```python
from build123d import *

# Parameters (mm, degrees)
ESQUISSE1_W              = 28
ESQUISSE1_H              = 28
BOSS_EXTRU_1_DEPTH       = 4
COQUE1_T                 = 1
ENL_V_MAT_EXTRU_1_REACH  = 43.449
ESQUISSE2_W              = 25
ESQUISSE2_H              = 15
CONG_1_R                 = 4
CONG_3_R                 = 1
ENL_V_MAT_EXTRU_13_REACH = 43.449
ESQUISSE21_W             = 12
ESQUISSE21_H             = 4
BOSS_EXTRU_8_START       = -15
BOSS_EXTRU_8_DEPTH       = 7
ESQUISSE26_W             = 12
ESQUISSE26_H             = 15
ENL_V_MAT_EXTRU_15_DEPTH = 4
BOSS_EXTRU_9_DEPTH       = 2
BOSS_EXTRU_9_DEPTH_BACK  = 1
ESQUISSE29_R             = 2
BOSS_EXTRU_10_DEPTH      = 2
BOSS_EXTRU_10_DEPTH_BACK = 1
ESQUISSE30_R             = 2


with BuildPart() as part:
    # Esquisse1 → Boss.-Extru.1 (new body)
    with BuildSketch(Plane.XY):
        with Locations((14, 14)):
            Rectangle(ESQUISSE1_W, ESQUISSE1_H)
    extrude(amount=BOSS_EXTRU_1_DEPTH)

    # Coque1
    coque1_openings = [part.faces().sort_by_distance(p)[0] for p in [
        (14, 0, 2),
    ]]
    offset(amount=COQUE1_T, openings=coque1_openings, kind=Kind.INTERSECTION)

    # Esquisse2 → Enlèv. mat.-Extru.1 (cut, up to next)
    with BuildSketch(Plane.XY.offset(5), mode=Mode.PRIVATE) as enl_v_mat_extru_1_sk1:
        with Locations((14, 11.5)):
            Rectangle(ESQUISSE2_W, ESQUISSE2_H)
    enl_v_mat_extru_1_tool1 = extrude(enl_v_mat_extru_1_sk1.sketch, amount=-ENL_V_MAT_EXTRU_1_REACH, mode=Mode.PRIVATE) & part.part
    add(enl_v_mat_extru_1_tool1.solids().sort_by_distance((14, 11.5, 5))[0], mode=Mode.SUBTRACT)

    # Congé1
    cong_1_edges = [part.edges().sort_by_distance(p)[0] for p in [
        (14, 29, -1),
    ]]
    fillet(cong_1_edges, radius=CONG_1_R)

    # Congé3
    cong_3_edges = [part.edges().sort_by_distance(p)[0] for p in [
        (26.5, 11.5, 5),
        (14, 19, 5),
        (1.5, 11.5, 5),
        (14, 4, 5),
    ]]
    fillet(cong_3_edges, radius=CONG_3_R - 0.0001)  # a hair under: the kernel refuses the full size

    # Esquisse21 → Enlèv. mat.-Extru.13 (cut, up to next)
    with BuildSketch(Plane(origin=(0, 0, -1), x_dir=(-1, 0, 0), z_dir=(0, 0, -1)), mode=Mode.PRIVATE) as enl_v_mat_extru_13_sk1:
        with Locations((-14, 2)):
            Rectangle(ESQUISSE21_W, ESQUISSE21_H)
    enl_v_mat_extru_13_tool1 = extrude(enl_v_mat_extru_13_sk1.sketch, amount=-ENL_V_MAT_EXTRU_13_REACH, mode=Mode.PRIVATE) & part.part
    add(enl_v_mat_extru_13_tool1.solids().sort_by_distance((14, 2, -1))[0], mode=Mode.SUBTRACT)

    # Esquisse24 → Boss.-Extru.8 (add, symmetric)
    with BuildSketch(Plane(origin=(29, 0, 0), x_dir=(0, 0, -1), z_dir=(1, 0, 0)).offset(BOSS_EXTRU_8_START)):
        with BuildLine():
            Line((1, 0), (17, 0))
            ThreePointArc((17, 0), (12.456832295, 12.328828006), (1, 18.761663039))
            Line((1, 18.761663039), (1, 0))
        make_face()
    extrude(amount=BOSS_EXTRU_8_DEPTH, both=True)

    # Esquisse26 → Enlèv. mat.-Extru.15 (cut)
    with BuildSketch(Plane.XZ):
        with Locations((14, -8.5)):
            Rectangle(ESQUISSE26_W, ESQUISSE26_H)
    extrude(amount=-ENL_V_MAT_EXTRU_15_DEPTH, mode=Mode.SUBTRACT)

    # Esquisse29 → Boss.-Extru.9 (add, two sides: drawn at the far end of the back side and taken through both)
    with BuildSketch(Plane(origin=(29, 0, 0), x_dir=(0, 0, -1), z_dir=(1, 0, 0)).offset(-BOSS_EXTRU_9_DEPTH_BACK)):
        with Locations((-2, 0)):
            Circle(ESQUISSE29_R)
    extrude(amount=BOSS_EXTRU_9_DEPTH + BOSS_EXTRU_9_DEPTH_BACK)

    # Esquisse30 → Boss.-Extru.10 (add, two sides: drawn at the far end of the back side and taken through both)
    with BuildSketch(Plane.ZY.offset(1).offset(-BOSS_EXTRU_10_DEPTH_BACK)):
        with Locations(Location((2, 0, 0), (0, 0, 180))):
            Circle(ESQUISSE30_R)
    extrude(amount=BOSS_EXTRU_10_DEPTH + BOSS_EXTRU_10_DEPTH_BACK)


solid = part.part
```
Check sheet for the modelled part. Datum: model origin and axes. Units: mm. A direction names the side the tool comes from. Give positions to 0.01 mm unless a question says otherwise; leave off trailing zeros. Write each loop counter-clockwise with the first axis right and the second up, starting at its lowest first coordinate (ties: lowest second). Pieces come first, ordered by that corner, then holes.
Item 1: Access from +Z, -Z, +X, -X, +Y, -Y to the whole of each face (thin tool, end or side, straight path). Record for faces 1 (the face through (14, 4, -8)), 2 (the face through (14, 21, -1)), 3 (the face through (-2, -2, 2)), 4 (the face through (7, 7, -7)), 5 (the face through (14.189, 19.301, 4.715)).
Item 2: Cross-section at B-B (z = -3). Enter the section's corners in (x, y), and give its area (3 significant figures).
Item 3: Scan lines: L1, parallel to Z at x = 1.5, y = 1.5; L2, parallel to X at y = 15, z = 1; L3, parallel to X at y = 1.5, z = -12. Record each from-to range of solid material in increasing order.
Item 4: Cross-section at D-D (z = -13.5). Enter the section's corners in (x, y).
Item 5: Draft check along X on faces 6 (the face through (7.4, 0, -7.8)), 7 (the face through (21, 7, -7)), 8 (the face through (28, 13, 2)). Enter one of: released by +X, released by -X, zero draft, split by the parting line, or undercut.
Item 6: Gauge pin test, flat ends, axial feed: pin 1 (8 mm diameter, centred on x = 15.5, z = -4.5, fed in from +Y); pin 2 (5 mm diameter, centred on y = 4, z = -6, fed in from +X); pin 3 (6 mm diameter, centred on x = 14.5, y = 22, fed in from -Z); pin 4 (10 mm diameter, centred on x = 27.5, z = -12, fed in from +Y). Record the tip position at first contact, or that the pin passes through.
Report:
1. face 1: -Y
1. face 2: -Z, +Y
1. face 3: -X
1. face 4: -Z, -X, +Y, -Y
1. face 5: +Z
2. outline: (7, 0) - (8, 0) - (8, 4) - (20, 4) - (20, 0) - (21, 0) - (21, 18.33) - (7, 18.33) - close
2. area: 209 mm2
3. L1: z = -1 to 0, 4 to 5
3. L2: x = -1 to 0, 28 to 29
3. L3: x = 7 to 8, 20 to 21
4. outline: (7, 0) - (8, 0) - (8, 4) - (20, 4) - (20, 0) - (21, 0) - (21, 10.99) - (7, 10.99) - close
5. face 6: zero draft
5. face 7: released by +X
5. face 8: undercut
6. pin 1: stops at y = 26.94
6. pin 2: stops at x = 21
6. pin 3: stops at z = -1
6. pin 4: passes through
